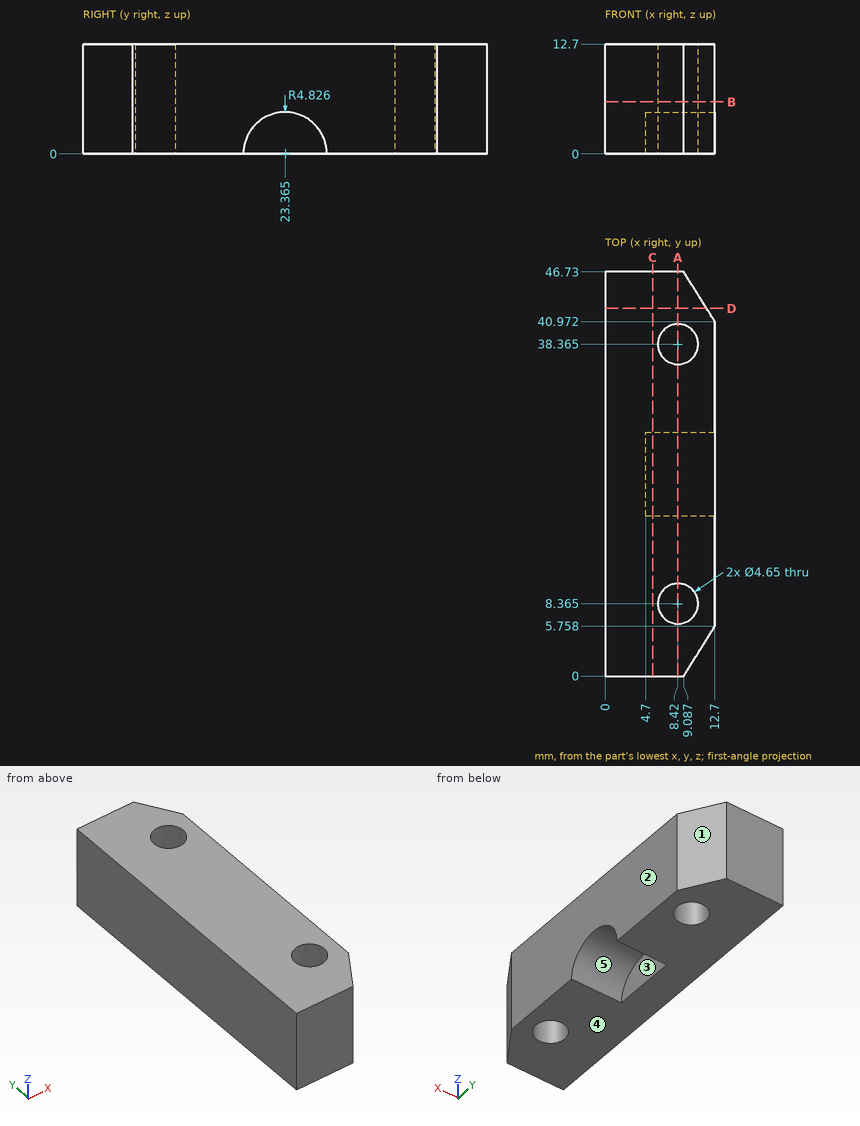
Study the drawing (mm; zero at the part's minimum x, y, z) and answer. A direction names the side the tool comes from. Coordinates: 2 decimals unless noted, no trailing zeros. Write each loop counter-clockwise with the first axis right and the second up, starting at its lowest first coordinate (ties: lowest second). Pieces come first, ordered by that corner, then holes. Notation, with made-up numbers: (25.25, 83) - (63.25, 83) arc R22 ccw to (63.25, 119) - close; hole circle Ø3 at (-10, -11.75). An arc over 180 degrees is marked (long way). One line per item, written item: value.
1) Find section D-D (y = 42.5). Give the vertices of the cut face in (x, z).
Geometry check:
outline: (0, 0) - (11.74, 0) - (11.74, 12.7) - (0, 12.7) - close
2) For a pull along Y with two mould halves and no side action, classify the marked faces 1, 2 and 3 as pulls with the +Y half, pulls with the -Y half, needs draft (parallel to the pull), parting line crosses it, or undercut.
Geometry check:
face 1: pulls with the +Y half
face 2: needs draft
face 3: undercut
3) Find section A-A (x = 8.42). Give the vertices of the cut face in (y, z) (1 decimal), and give its area (3 significant figures).
Geometry check:
outline: (0, 0) - (6, 0) - (6, 12.7) - (0, 12.7) - close; (10.7, 0) - (18.5, 0) arc R4.8 cw to (28.2, 0) - (36, 0) - (36, 12.7) - (10.7, 12.7) - close; (40.7, 0) - (46.7, 0) - (46.7, 12.7) - (40.7, 12.7) - close
area: 439 mm2
4) This flat-tipped pin is pushed along its axis until it touches: pin 1 Ø1.4 at (y, z) = (23.5, 2.5) entering from +X. Where does it stop, or does it pass through?
Geometry check:
pin 1: stops at x = 4.7
5) A tool of negligible diameter and unlimited length cuts with its end or side. For the marked faces 4 and 5, from which of +Z, -Z, +X, -X, +Y, -Y can it reach the whole face along a straight path? Write none if from no direction.
Geometry check:
face 4: -Z, +X, -X, +Y, -Y
face 5: -Z, +X
6) Consider line 1 along Y through (x, z) = (8.42, 8); line 2 along Y through (x, z) = (7.5, 8.5); line 3 along Y through (x, z) = (8.42, 3.75) (1 decimal). Determine where each line is inside the solid, lowest interval first. Write a range as from..to.
Geometry check:
line 1: y = 0..6.04, 10.69..36.04, 40.69..46.73
line 2: y = 0..6.23, 10.5..36.23, 40.5..46.73
line 3: y = 0..6, 10.7..20.3, 26.4..36, 40.7..46.7
7) Find section C-C (x = 5.5). Give the vertices of the cut face in (y, z) (1 decimal).
Geometry check:
outline: (0, 0) - (18.5, 0) arc R4.8 cw to (28.2, 0) - (46.7, 0) - (46.7, 12.7) - (0, 12.7) - close
8) Find section B-B (z = 6). Count the separate pieces of the cut face and the enclosed holes in it, and give its area (3 significant figures).
Geometry check:
separate pieces: 1
enclosed holes: 2
area: 539 mm2
